```python
from build123d import *

# Parameters (mm, degrees)
PAD_DEPTH    = 88
PAD001_DEPTH = 55
CHAMFER_SIZE = 10


with BuildPart() as part:
    # Sketch → Pad (new body)
    with BuildSketch(Plane.XY):
        with BuildLine():
            ThreePointArc((-47, 0), (-24, -23), (-1, 0))
            Line((-1, 0), (0, 0))
            Line((0, 0), (0, -15))
            Line((0, -15), (32.5, -15))
            Line((32.5, -15), (32.5, 0))
            Line((32.5, 0), (42.5, 0))
            Line((42.5, 0), (42.5, -35))
            Line((22.5, -35), (42.5, -35))
            Line((22.5, -30), (22.5, -35))
            Line((-37, -30), (22.5, -30))
            Line((-37, -35), (-37, -30))
            Line((-57, -35), (-37, -35))
            Line((-57, -35), (-57, 0))
            Line((-57, 0), (-47, 0))
        make_face()
    extrude(amount=PAD_DEPTH)

    # Sketch001 (on Face16 of Pad) → Pad001 (join)
    with BuildSketch(Plane.XY.offset(88)):
        Polygon((0, -23), (42.5, -23), (42.5, -35), (22.5, -35), (22.5, -30), (0, -30), align=None)
    extrude(amount=PAD001_DEPTH)

    # Chamfer
    chamfer_edges = [part.edges().sort_by_distance(p)[0] for p in [
        (0, -26.5, 143),
        (42.5, -29, 143),
    ]]
    chamfer(chamfer_edges, length=CHAMFER_SIZE)


solid = part.part
```
Can you work these out from the model? Positions are in its coordinate system, mm. A direction names the side the tool comes from. Give positions to 0.01 mm unless a question says otherwise; leave off trailing zeros. Order: outer loops, then holes, each group sorted by start corner. A loop starts at its lowest first (then second) coordinate and runs counter-clockwise, first axis right, second up. Notation, with made-up numbers: M -23.5,-38 L 18.5,-38 A31 ccw 18.5,1 Z; hole C 82,1.5 d2. An arc over 180 degrees is marked long. One line per item, written item: value.
1) I want a section at B-B, the plane z = 27.5. List the corners of the cut face in (x, y) for me.
Answer sheet:
outline: M -57,-35 L -37,-35 L -37,-30 L 22.5,-30 L 22.5,-35 L 42.5,-35 L 42.5,0 L 32.5,0 L 32.5,-15 L 0,-15 L 0,0 L -1,0 A23 cw -47,0 L -57,0 Z
2) Please list where these lines run through material, in increasing order: line 1 along X through (y, z) = (-31, 79); line 2 along X through (y, z) = (-12, 23.5); line 3 along X through (y, z) = (-13.5, 54).
Answer sheet:
line 1: x = -57 to -37, 22.5 to 42.5
line 2: x = -57 to -43.62, -4.38 to 0, 32.5 to 42.5
line 3: x = -57 to -42.62, -5.38 to 0, 32.5 to 42.5
3) I want a section at D-D, the plane x = 6.5. List the corners of the cut face in (y, z) for me.
Answer sheet:
outline: M -30,0 L -15,0 L -15,88 L -23,88 L -23,139.5 L -30,139.5 Z
4) On a 3-axis mill with a long thin cutter (end or side, diameter ignored), from which of +Z, -Z, +X, -X, +Y, -Y can I reach the whole of each face in a straight line? I mean faces 1 (the face through (5, -27, 138)), 2 (the face through (21, -23, 115)), 3 (the face through (-7, -30, 55)), 4 (the face through (16, -15, 43)). Say none if no direction works.
Answer sheet:
face 1: +Z, -X, +Y, -Y
face 2: +Z, +X, -X, +Y
face 3: +Z, -Z, -Y
face 4: +Z, -Z, +Y
5) For P1, Ø21, axis at x = 14.5, z = 114, coming from the +Y side; P2, Ø18, axis at x = -16.5, z = 83, coming from the -Y side; P3, Ø2, axis at y = -26, z = 119, coming from the -X side; P4, Ø17.5, axis at x = -19.5, y = -9, coming from the +Z side, each with a flat end and sliding along its axis, tell me the tip position at first contact or that it passes through.
Answer sheet:
P1: stops at y = -23
P2: stops at y = -30
P3: stops at x = 0
P4: passes through
6) I want a section at C-C, the plane y = -27. List the corners of the cut face in (x, z) for me, plus the area to 3 significant figures.
Answer sheet:
outline: M -57,0 L 42.5,0 L 42.5,133 L 32.5,143 L 10,143 L 0,133 L 0,88 L -57,88 Z
area: 11,000 mm^2
7) We'd pull the mould along X, two halves only. Please class faces 5 (the face through (37.6, -28.9, 137.9)), 6 (the face through (24, -28, 143)), 7 (the face through (-37, -33, 43)), 8 (the face through (32.5, -8, 43)): released by +X, released by -X, zero draft, split by the parting line, or undercut.
Answer sheet:
face 5: released by +X
face 6: zero draft
face 7: undercut
face 8: undercut
8) I want a section at A-A, the plane y = -2.5. List the corners of the cut face in (x, z) for me.
Answer sheet:
outline: M -57,0 L -46.86,0 L -46.86,88 L -57,88 Z; M -1.14,0 L 0,0 L 0,88 L -1.14,88 Z; M 32.5,0 L 42.5,0 L 42.5,88 L 32.5,88 Z
